Work out the finished part from the listing and answer in its coordinate system (mm). Face numbers are marked on the shaded views. Round coordinates to 2 decimals unless told otherwise and drop trailing zeros. Loops run counter-clockwise (first coordinate to the right, second up) from the corner with the lowest first, then second, coordinate; pieces in that order, holes last. Notation, with made-up numbers: M 28,75.25 L 80,75.25 A27 cw 80,103.25 Z; hole C -13.75,35 d1. An arc over 180 degrees is marked long. One line per item, written item: value.
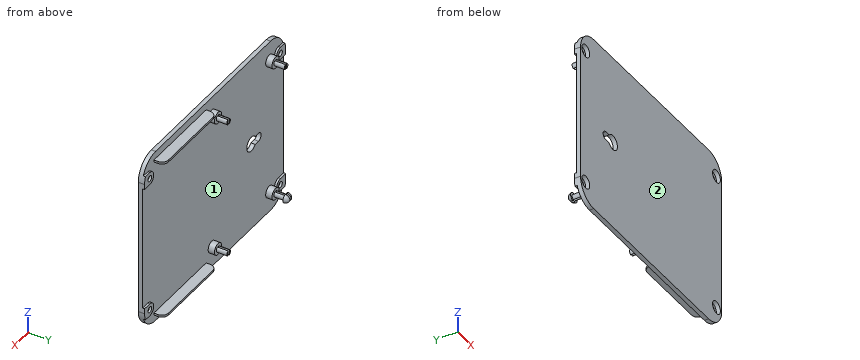
```python
from build123d import *

# Parameters (mm, degrees)
BOSS_EXTRUDE2_DEPTH = 2
CUT_EXTRUDE2_DEPTH  = 7
SKETCH10_W          = 40
SKETCH10_H          = 1
BOSS_EXTRUDE3_DEPTH = 7
CUT_EXTRUDE4_DEPTH  = 1
CUT_EXTRUDE5_DEPTH  = 1
SKETCH14_R          = 1.375
BOSS_EXTRUDE4_DEPTH = 10
SKETCH15_R          = 2.75
BOSS_EXTRUDE5_DEPTH = 5
BOSS_EXTRUDE8_DEPTH = 3
SKETCH21_R          = 3
CUT_EXTRUDE7_DEPTH  = 1.9
SKETCH22_R          = 1.4
CUT_EXTRUDE8_DEPTH  = 15
SKETCH24_W          = 1
SKETCH24_H          = 3.418232964
SKETCH24_H_2        = 3.173713674
SKETCH24_H_3        = 3.19842194
CUT_EXTRUDE10_DEPTH = 5
REVOLVE1_ANGLE      = 180
REVOLVE2_ANGLE      = 180


with BuildPart() as part:
    # Sketch3 → Boss-Extrude2 (new body)
    with BuildSketch(Plane(origin=(0, 0, 0), x_dir=(1, 0, 0), z_dir=(0, 1, 0))):
        with BuildLine():
            Line((-30.001043465, -34.015189653), (57.998956535, -34.015189653))
            ThreePointArc((57.998956535, -34.015189653), (65.070024347, -31.086257464), (67.998956535, -24.015189653))
            Line((67.998956535, -24.015189653), (67.998956535, 40.984810347))
            ThreePointArc((67.998956535, 40.984810347), (65.070024347, 48.055878159), (57.998956535, 50.984810347))
            Line((57.998956535, 50.984810347), (-30.001043465, 50.984810347))
            ThreePointArc((-30.001043465, 50.984810347), (-37.072111277, 48.055878159), (-40.001043465, 40.984810347))
            Line((-40.001043465, 40.984810347), (-40.001043465, -24.015189653))
            ThreePointArc((-40.001043465, -24.015189653), (-37.072111277, -31.086257464), (-30.001043465, -34.015189653))
        make_face()
    extrude(amount=BOSS_EXTRUDE2_DEPTH)

    # Sketch6 → Cut-Extrude2 (cut)
    with BuildSketch(Plane(origin=(0, 2, 0), x_dir=(1, 0, 0), z_dir=(0, 1, 0))):
        with BuildLine():
            Line((-18.182060551, 10.483778137), (-20.721753803, 10.483778137))
            ThreePointArc((-20.721753803, 10.483778137), (-22.720721593, 8.484810347), (-20.721753803, 6.485842558))
            Line((-20.721753803, 6.485842558), (-18.182060551, 6.485842558))
            ThreePointArc((-18.182060551, 6.485842558), (-11.809060764, 8.484810347), (-18.182060551, 10.483778137))
        make_face()
    extrude(amount=-CUT_EXTRUDE2_DEPTH, mode=Mode.SUBTRACT)

    # Sketch10 → Boss-Extrude3 (add)
    with BuildSketch(Plane(origin=(0, 0, 0), x_dir=(1, 0, 0), z_dir=(0, 1, 0))):
        with Locations((39.263184903, 46.984810347)):
            Rectangle(SKETCH10_W, SKETCH10_H)
        with Locations((39.263184903, -30.015189653)):
            Rectangle(SKETCH10_W, SKETCH10_H)
    extrude(amount=BOSS_EXTRUDE3_DEPTH)

    # Sketch12 → Cut-Extrude4 (cut)
    with BuildSketch(Plane.XY.offset(30.515189653)):
        with BuildLine():
            Line((56.263184903, 7), (59.263184903, 7))
            Line((59.263184903, 7), (59.263184903, 4))
            ThreePointArc((59.263184903, 4), (58.384505246, 6.121320344), (56.263184903, 7))
        make_face()
        with BuildLine():
            Line((19.263184903, 4), (19.263184903, 7))
            Line((19.263184903, 7), (22.263184903, 7))
            ThreePointArc((22.263184903, 7), (20.141864559, 6.121320344), (19.263184903, 4))
        make_face()
    extrude(amount=-CUT_EXTRUDE4_DEPTH, mode=Mode.SUBTRACT)

    # Sketch13 → Cut-Extrude5 (cut)
    with BuildSketch(Plane(origin=(0, 0, -47.484810347), x_dir=(-1, 0, 0), z_dir=(0, 0, -1))):
        with BuildLine():
            Line((-56.263184903, 7), (-59.263184903, 7))
            Line((-59.263184903, 7), (-59.263184903, 4))
            ThreePointArc((-59.263184903, 4), (-58.384505246, 6.121320344), (-56.263184903, 7))
        make_face()
        with BuildLine():
            Line((-19.263184903, 4), (-19.263184903, 7))
            Line((-19.263184903, 7), (-22.263184903, 7))
            ThreePointArc((-22.263184903, 7), (-20.141864559, 6.121320344), (-19.263184903, 4))
        make_face()
    extrude(amount=-CUT_EXTRUDE5_DEPTH, mode=Mode.SUBTRACT)

    # Sketch14 → Boss-Extrude4 (add)
    with BuildSketch(Plane.XZ):
        with Locations(Location((-29.011006112, 25.011760646, 0), (0, 0, 270))):
            Circle(SKETCH14_R)
        with Locations(Location((14.981881874, 25.011760646, 0), (0, 0, 270))):
            Circle(SKETCH14_R)
        with Locations(Location((14.981881874, -40.988239354, 0), (0, 0, 270))):
            Circle(SKETCH14_R)
        with Locations(Location((-29.011006112, -40.988239354, 0), (0, 0, 270))):
            Circle(SKETCH14_R)
    extrude(amount=-BOSS_EXTRUDE4_DEPTH)

    # Sketch15 → Boss-Extrude5 (add)
    with BuildSketch(Plane.XZ):
        with Locations(Location((-29.011006112, 25.011760646, 0), (0, 0, 270))):
            Circle(SKETCH15_R)
        with Locations(Location((14.981881874, 25.011760646, 0), (0, 0, 270))):
            Circle(SKETCH15_R)
        with Locations(Location((14.981881874, -40.988239354, 0), (0, 0, 270))):
            Circle(SKETCH15_R)
        with Locations(Location((-29.011006112, -40.988239354, 0), (0, 0, 270))):
            Circle(SKETCH15_R)
    extrude(amount=-BOSS_EXTRUDE5_DEPTH)

    # Sketch5 → Boss-Extrude8 (add)
    with BuildSketch(Plane(origin=(0, 0, 34.015189653), x_dir=(1, 0, 0), z_dir=(0, 1, 0))):
        with BuildLine():
            Line((-36.001043465, 78.5), (-39.368540462, 78.5))
            ThreePointArc((-39.368540462, 78.5), (-39.841647358, 76.778346145), (-40.001043465, 75))
            Line((-40.001043465, 75), (-40.001043465, 72.5))
            Line((-40.001043465, 72.5), (-36.001043465, 72.5))
            ThreePointArc((-36.001043465, 72.5), (-33.001043465, 75.5), (-36.001043465, 78.5))
        make_face()
        with BuildLine():
            Line((63.998956535, 78.5), (67.366453533, 78.5))
            ThreePointArc((67.366453533, 78.5), (67.839560429, 76.778346145), (67.998956535, 75))
            Line((67.998956535, 75), (67.998956535, 72.5))
            Line((67.998956535, 72.5), (63.998956535, 72.5))
            ThreePointArc((63.998956535, 72.5), (60.998956535, 75.5), (63.998956535, 78.5))
        make_face()
        with BuildLine():
            Line((63.998956535, 12.5), (67.998956535, 12.5))
            Line((67.998956535, 12.5), (67.998956535, 10))
            ThreePointArc((67.998956535, 10), (67.839560429, 8.221653855), (67.366453533, 6.5))
            Line((67.366453533, 6.5), (63.998956535, 6.5))
            ThreePointArc((63.998956535, 6.5), (60.998956535, 9.5), (63.998956535, 12.5))
        make_face()
        with BuildLine():
            Line((-36.001043465, 12.5), (-40.001043465, 12.5))
            Line((-40.001043465, 12.5), (-40.001043465, 10))
            ThreePointArc((-40.001043465, 10), (-39.841647358, 8.221653855), (-39.368540462, 6.5))
            Line((-39.368540462, 6.5), (-36.001043465, 6.5))
            ThreePointArc((-36.001043465, 6.5), (-33.001043465, 9.5), (-36.001043465, 12.5))
        make_face()
    extrude(amount=BOSS_EXTRUDE8_DEPTH)

    # Sketch21 → Cut-Extrude7 (cut)
    with BuildSketch(Plane.XZ):
        with Locations(Location((-36.001043465, 24.515189653, 0), (0, 0, 270))):
            Circle(SKETCH21_R)
        with Locations(Location((63.998956535, 24.515189653, 0), (0, 0, 270))):
            Circle(SKETCH21_R)
        with Locations(Location((63.998956535, -41.484810347, 0), (0, 0, 270))):
            Circle(SKETCH21_R)
        with Locations(Location((-36.001043465, -41.484810347, 0), (0, 0, 270))):
            Circle(SKETCH21_R)
    extrude(amount=-CUT_EXTRUDE7_DEPTH, mode=Mode.SUBTRACT)

    # Sketch22 → Cut-Extrude8 (cut)
    with BuildSketch(Plane.XZ.offset(-1.9)):
        with Locations(Location((-36.001043465, 24.515189653, 0), (0, 0, 270))):
            Circle(SKETCH22_R)
        with Locations(Location((63.998956535, 24.515189653, 0), (0, 0, 270))):
            Circle(SKETCH22_R)
        with Locations(Location((63.998956535, -41.484810347, 0), (0, 0, 270))):
            Circle(SKETCH22_R)
        with Locations(Location((-36.001043465, -41.484810347, 0), (0, 0, 270))):
            Circle(SKETCH22_R)
    extrude(amount=-CUT_EXTRUDE8_DEPTH, mode=Mode.SUBTRACT)

    # Sketch24 → Cut-Extrude10 (cut)
    with BuildSketch(Plane(origin=(0, 10, 0), x_dir=(1, 0, 0), z_dir=(0, 1, 0))):
        with Locations((-29.011006112, 40.988239354)):
            Rectangle(SKETCH24_W, SKETCH24_H)
        with Locations((14.981881874, 40.988239354)):
            Rectangle(SKETCH24_W, SKETCH24_H_2)
        with Locations((14.981881874, -25.011760646)):
            Rectangle(SKETCH24_W, SKETCH24_H_3)
        with Locations((-29.011006112, -25.011760646)):
            Rectangle(SKETCH24_W, SKETCH24_H_3)
    extrude(amount=-CUT_EXTRUDE10_DEPTH, mode=Mode.SUBTRACT)

    # Sketch27 → Revolve1 (revolve)
    with BuildSketch(Plane(origin=(-29.511006112, 0, 0), x_dir=(0, 0, -1), z_dir=(1, 0, 0))):
        with BuildLine():
            Line((40.988239354, 10), (42.988239354, 10))
            add(Edge.make_bspline(
                [(42.988239354, 10), (42.701903719, 11.805725315), (40.988239354, 12.142709999)],
                knots=[0, 0, 0, 1, 1, 1], degree=2))
            Line((40.988239354, 12.142709999), (40.988239354, 10))
        make_face()
    revolve(axis=Axis((-29.511006112, 10, -40.988239354), (0, 1, 0)), revolution_arc=REVOLVE1_ANGLE)

    # Sketch28 → Revolve2 (revolve)
    with BuildSketch(Plane.ZY.offset(28.511006112)):
        with BuildLine():
            add(Edge.make_bspline(
                [(-38.988239352, 9.999999987), (-39.274574983, 11.805725311), (-40.98823935, 12.142709998)],
                knots=[0, 0, 0, 1, 1, 1], degree=2))
            Line((-40.98823935, 12.142709998), (-40.988239354, 10))
            Line((-40.988239354, 9.999999993), (-39.707370508, 9.999999989))
            Line((-39.707370508, 9.999999989), (-38.988239352, 9.999999987))
        make_face()
    revolve(axis=Axis((-28.511006112, 12.142709998, -40.98823935), (0, 1.0, 2.1018108519828045e-09)), revolution_arc=REVOLVE2_ANGLE)


solid = part.part
```
1) Find section A-A (z = -8). Give the vertices of the cut face in (x, y), then the cut area to 3 significant figures.
Check values:
outline: M -40,0 L -22.66,0 L -22.66,2 L -40,2 Z; M -11.84,0 L 68,0 L 68,2 L -11.84,2 Z
area: 194 mm2
2) Find the intervals of material crossed by probe 1 along Z at (x, y) = (22, 3.75); probe 2 along Y at (x, z) = (-31, -29); probe 3 along X at (y, z) = (8.5, 26), in increasing order. Write a range as from..to.
Check values:
probe 1: -47.48..-46.48, 29.52..30.52
probe 2: 0..2
probe 3: -29.97..-29.51, -28.51..-28.05, 14.03..14.48, 15.48..15.94
3) The mould has two halves that part along Z. Classify the marked faces 1 and 2: +Z half, -Z half, draft (parallel to the pull), parting line (faces both ways), or undercut.
Check values:
face 1: undercut
face 2: draft
4) Find section B-B (x = 33). Give the vertices of the cut face in (y, z), then the cut area to 3 significant figures.
Check values:
outline: M 0,-50.98 L 2,-50.98 L 2,-47.48 L 7,-47.48 L 7,-46.48 L 2,-46.48 L 2,29.52 L 7,29.52 L 7,30.52 L 2,30.52 L 2,34.02 L 0,34.02 Z
area: 180 mm2
5) Find section C-C (x = -9.5). Give the vertices of the cut face in (y, z), then the cut area to 3 significant figures.
Check values:
outline: M 0,-50.98 L 2,-50.98 L 2,34.02 L 0,34.02 Z
area: 170 mm2
6) Each of these flat-tipped pins is pushed along its axis until it touches: pin 1 (1.1 mm diameter, centred on y = 3, z = 30, fed in from -X); pin 2 (6 mm diameter, centred on x = -29.5, z = -40.5, fed in from +Y); pin 3 (4.5 mm diameter, centred on x = 15, z = 26, fed in from +Y); pin 4 (9.5 mm diameter, centred on x = -36, z = 24.52, fed in from +Y). Where does it stop, or does it pass through?
Check values:
pin 1: x = 19.26
pin 2: y = 12.14
pin 3: y = 10
pin 4: y = 5
